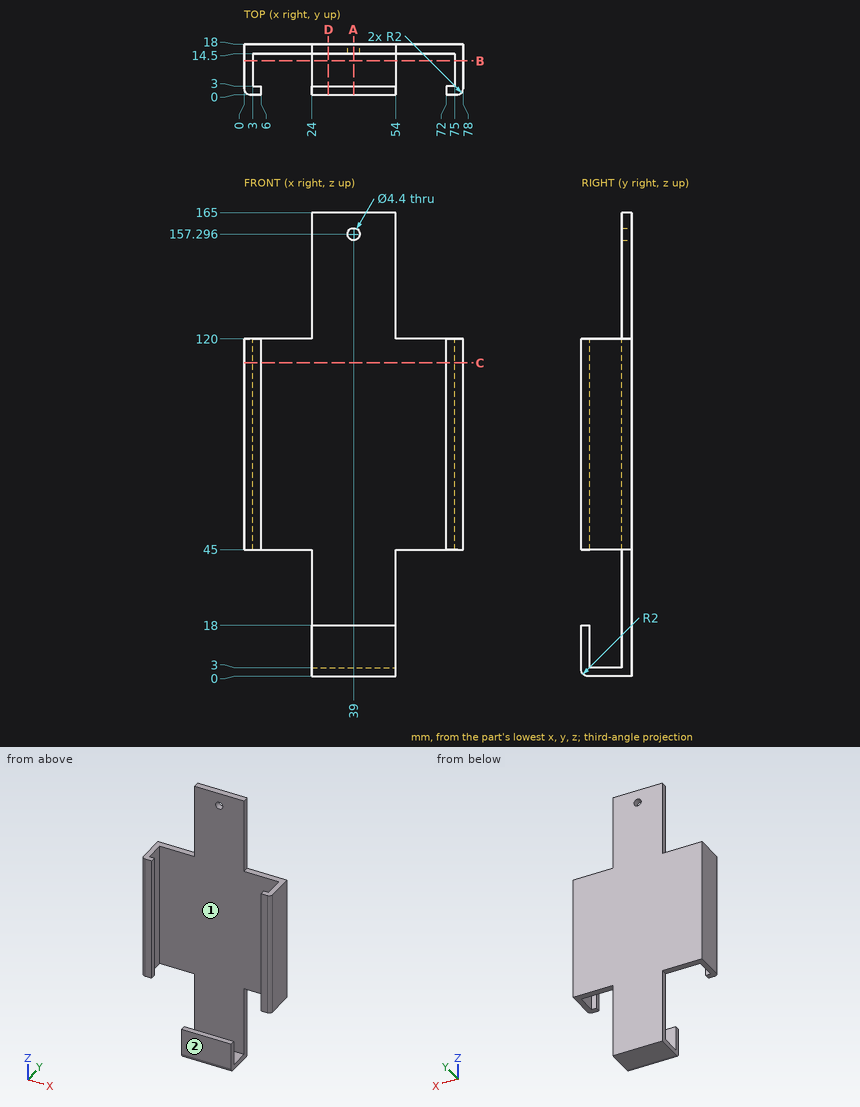
Can you work these out from the drawing? Everything is in mm from the part's minimum corner. Give positions to 0.01 mm unless a question says otherwise; leave off trailing zeros. Order: outer loops, then holes, each group sorted by start corner. A loop starts at its lowest first (then second) coordinate and runs counter-clockwise, first axis right, second up. Notation, with made-up numbers: M 9,-13.75 L 57,-13.75 A10 ccw 57,1.25 Z; hole C -34,-38 d9. An arc over 180 degrees is marked long. One line per item, written item: value.
Item 1: If we section it at C-C on z = 111.5: Write out the boundary of the cut face in (x, y).
Verdict:
outline: M 0,2 A2 ccw 2,0 L 6,0 L 6,3 L 3,3 L 3,14.5 L 75,14.5 L 75,3 L 72,3 L 72,0 L 76,0 A2 ccw 78,2 L 78,18 L 0,18 Z
Item 2: If we section it at B-B on y = 12: Write out the boundary of the cut face in (x, z), and give its area (3 significant figures).
Verdict:
outline: M 0,45 L 3,45 L 3,120 L 0,120 Z; M 24,0 L 54,0 L 54,3 L 24,3 Z; M 75,45 L 78,45 L 78,120 L 75,120 Z
area: 540 mm2
Item 3: For pin 1 (8 mm diameter, centred on x = 23, z = 41, fed in from -Y); pin 2 (1.8 mm diameter, centred on y = 16.5, z = 152, fed in from -X); pin 3 (1 mm diameter, centred on y = 16, z = 142.5, fed in from +X), each with a flat end and sliding along its axis, tell me the tip position at first contact or that it passes through.
Verdict:
pin 1: y = 14.5
pin 2: x = 24
pin 3: x = 54
Item 4: If we section it at A-A on x = 39: Write out the boundary of the cut face in (y, z).
Verdict:
outline: M 0,2 A2 ccw 2,0 L 18,0 L 18,155.1 L 14.5,155.1 L 14.5,3 L 3,3 L 3,18 L 0,18 Z; M 14.5,159.5 L 18,159.5 L 18,165 L 14.5,165 Z
Item 5: Please list where these lines run through material, in increasing order: line 1 (Z direction, x = 39, y = 16.3); line 2 (X direction, y = 2.75, z = 91); line 3 (X direction, y = 9.5, z = 80).
Verdict:
line 1: 0 to 155.1, 159.5 to 165
line 2: 0 to 6, 72 to 78
line 3: 0 to 3, 75 to 78
Item 6: If we mould it in two halves opening along X, with no side actions, what happens to the marked faces 1 and 2? For each: pulls with the +X half, pulls with the -X half, needs draft (parallel to the pull), parting line crosses it, or undercut.
Verdict:
face 1: undercut
face 2: needs draft
Item 7: If we section it at D-D on x = 30: Write out the boundary of the cut face in (y, z).
Verdict:
outline: M 0,2 A2 ccw 2,0 L 18,0 L 18,165 L 14.5,165 L 14.5,3 L 3,3 L 3,18 L 0,18 Z
